```python
from build123d import *

# Parameters (mm, degrees)
BOSS_EXTRUDE1_DEPTH = 6.35


with BuildPart() as part:
    # Sketch1 → Boss-Extrude1 (new body)
    with BuildSketch(Plane.XY):
        Polygon((0, 0), (12.573, 0), (12.573, 6.35), (25.527, 6.35), (25.527, 0), (101.6, 0), (101.6, -127.635), (127.0635, -127.635), (127.0635, -133.985), (139.6365, -133.985), (139.6365, -127.635), (152.4635, -127.635), (152.4635, -133.985), (165.0365, -133.985), (165.0365, -127.635), (190.5, -127.635), (190.5, 0), (266.573, 0), (266.573, 6.35), (279.527, 6.35), (279.527, 0), (292.1, 0), (292.1, -12.827), (285.75, -12.827), (285.75, -25.273), (292.1, -25.273), (292.1, -38.227), (285.75, -38.227), (285.75, -50.673), (292.1, -50.673), (292.1, -63.627), (285.75, -63.627), (285.75, -76.073), (292.1, -76.073), (292.1, -89.027), (285.75, -89.027), (285.75, -101.473), (292.1, -101.473), (292.1, -114.427), (285.75, -114.427), (285.75, -126.873), (292.1, -126.873), (292.1, -139.827), (285.75, -139.827), (285.75, -152.273), (292.1, -152.273), (292.1, -165.227), (285.75, -165.227), (285.75, -177.673), (292.1, -177.673), (292.1, -190.627), (285.75, -190.627), (285.75, -203.073), (292.1, -203.073), (292.1, -216.027), (285.75, -216.027), (285.75, -228.473), (292.1, -228.473), (292.1, -241.427), (285.75, -241.427), (285.75, -253.873), (292.1, -253.873), (292.1, -266.827), (285.75, -266.827), (285.75, -279.273), (292.1, -279.273), (292.1, -292.227), (285.75, -292.227), (285.75, -304.673), (292.1, -304.673), (292.1, -317.627), (285.75, -317.627), (285.75, -330.073), (292.1, -330.073), (292.1, -342.9), (279.273, -342.9), (279.273, -336.55), (266.827, -336.55), (266.827, -222.25), (25.273, -222.25), (25.273, -336.55), (12.827, -336.55), (12.827, -342.9), (0, -342.9), (0, -330.073), (6.35, -330.073), (6.35, -317.627), (0, -317.627), (0, -304.673), (6.35, -304.673), (6.35, -292.227), (0, -292.227), (0, -279.273), (6.35, -279.273), (6.35, -266.827), (0, -266.827), (0, -253.873), (6.35, -253.873), (6.35, -241.427), (0, -241.427), (0, -228.473), (6.35, -228.473), (6.35, -216.027), (0, -216.027), (0, -203.073), (6.35, -203.073), (6.35, -190.627), (0, -190.627), (0, -177.673), (6.35, -177.673), (6.35, -165.227), (0, -165.227), (0, -152.273), (6.35, -152.273), (6.35, -139.827), (0, -139.827), (0, -126.873), (6.35, -126.873), (6.35, -114.427), (0, -114.427), (0, -101.473), (6.35, -101.473), (6.35, -89.027), (0, -89.027), (0, -76.073), (6.35, -76.073), (6.35, -63.627), (0, -63.627), (0, -50.673), (6.35, -50.673), (6.35, -38.227), (0, -38.227), (0, -25.273), (6.35, -25.273), (6.35, -12.827), (0, -12.827), align=None)
        Polygon((260.870458318, -155.351665797), (248.363399855, -157.556997654), (247.842941537, -154.605331856), (260.35, -152.4), align=None, mode=Mode.SUBTRACT)
        Polygon((235.856341392, -159.76232951), (223.349282928, -161.967661366), (222.82882461, -159.015995569), (235.335883073, -156.810663713), align=None, mode=Mode.SUBTRACT)
        Polygon((210.842224465, -164.172993223), (198.335166002, -166.378325079), (197.814707684, -163.426659282), (210.321766147, -161.221327425), align=None, mode=Mode.SUBTRACT)
        Polygon((185.828107539, -168.583656936), (173.321049075, -170.788988792), (172.800590757, -167.837322995), (185.30764922, -165.631991138), align=None, mode=Mode.SUBTRACT)
        Polygon((160.813990612, -172.994320648), (148.306932149, -175.199652505), (147.786473831, -172.247986707), (160.293532294, -170.042654851), align=None, mode=Mode.SUBTRACT)
        Polygon((135.799873686, -177.404984361), (123.292815222, -179.610316217), (122.772356904, -176.65865042), (135.279415367, -174.453318564), align=None, mode=Mode.SUBTRACT)
        Polygon((110.785756759, -181.815648074), (98.278698296, -184.02097993), (97.758239978, -181.069314133), (110.265298441, -178.863982276), align=None, mode=Mode.SUBTRACT)
    extrude(amount=BOSS_EXTRUDE1_DEPTH)


solid = part.part
```
The listing builds one solid part. Answer for the finished solid, in the listing's coordinates (mm). Give positions to 0.01 mm unless a question says otherwise; leave off trailing zeros. Loops run counter-clockwise (first coordinate to the right, second up) from the corner with the lowest first, then second, coordinate; pieces in that order, holes last. Notation, with made-up numbers: (-18.5, -38) - (-13.5, -38) arc R16 ccw to (-13.5, -21) - close; hole circle Ø3 at (61.5, 36.5). An arc over 180 degrees is marked (long way). Answer as CSV lines item,"result". Start each with the question number.
Item 1: A cutting plane is placed at D-D on x = 29.5. Determine the outline of the cut face in (y, z), then the cut area to 3 significant figures.
Item 2: A cutting plane is placed at C-C on z = 4.25. Count the separate pieces of the cut face and the enclosed holes in it, then the cut area to 3 significant figures.
Item 3: A cutting plane is placed at B-B on x = 180.5. Determine the outline of the cut face in (y, z) (3 decimals), then the cut area to 3 significant figures.
Item 4: Each of these flat-tipped pins is pushed along its axis until it touches: pin 1 (1.9 mm diameter, centred on x = 151, z = 3.5, fed in from -Y); pin 2 (3 mm diameter, centred on x = 4.5, z = 3, fed in from +Y); pin 3 (3 mm diameter, centred on y = -223, z = 4.5, fed in from -X). Where does it stop, or does it pass through?
Item 5: A cutting plane is placed at A-A on y = -70.5. Determine the outline of the cut face in (x, z).
Item 6: Find the intervals of material crossed by line 1 (X direction, y = -29.5, z = 5.5); line 2 (X direction, y = -44, z = 3.25); line 3 (Y direction, x = 271, z = 1.75), in increasing order. Write a range as from..to.
Found:
1,outline,"(-222.25, 0) - (0, 0) - (0, 6.35) - (-222.25, 6.35) - close"
1,area,"1,410 mm^2"
2,separate pieces,"1"
2,enclosed holes,"7"
2,area,"57,200 mm^2"
3,outline,"(-222.25, 0) - (-169.523, 0) - (-169.523, 6.35) - (-222.25, 6.35) - close; (-166.48, 0) - (-127.635, 0) - (-127.635, 6.35) - (-166.48, 6.35) - close"
3,area,"581 mm^2"
4,pin 1,"stops at y = -222.25"
4,pin 2,"stops at y = 0"
4,pin 3,"stops at x = 6.35"
5,outline,"(6.35, 0) - (101.6, 0) - (101.6, 6.35) - (6.35, 6.35) - close; (190.5, 0) - (285.75, 0) - (285.75, 6.35) - (190.5, 6.35) - close"
6,line 1,"x = 0..101.6, 190.5..292.1"
6,line 2,"x = 6.35..101.6, 190.5..285.75"
6,line 3,"y = -336.55..6.35"
